Check sheet for the modelled part. Datum: model origin and axes. Units: mm. A direction names the side the tool comes from. Round coordinates to 2 decimals unless told otherwise and drop trailing zeros. Write each loop counter-clockwise with the first axis right and the second up, starting at its lowest first coordinate (ties: lowest second). Pieces come first, ordered by that corner, then holes. Notation, with made-up numbers: (59, 27) -> (75, 27) arc R23 cw to (75, 64) -> close; hole circle Ø6 at (71, 79.5). An arc over 180 degrees is marked (long way). Put each result on its own line as item: value. Start each with the question number.
from build123d import *

# Parameters (mm, degrees)
SKETCH1_W           = 5
SKETCH1_H           = 128.5
BOSS_EXTRUDE1_DEPTH = 2
CUT_EXTRUDE1_DEPTH  = 2.54
FILLET1_R           = 1.27


with BuildPart() as part:
    # Sketch1 → Boss-Extrude1 (new body)
    with BuildSketch(Plane.XY):
        Rectangle(SKETCH1_W, SKETCH1_H)
        with BuildLine():
            Line((-0.254, -59.6), (0.254, -59.6))
            ThreePointArc((0.254, -59.6), (1.904, -61.25), (0.254, -62.9))
            Line((0.254, -62.9), (-0.254, -62.9))
            ThreePointArc((-0.254, -62.9), (-1.904, -61.25), (-0.254, -59.6))
        make_face(mode=Mode.SUBTRACT)
        with BuildLine():
            Line((-0.254, 62.9), (0.254, 62.9))
            ThreePointArc((0.254, 62.9), (1.904, 61.25), (0.254, 59.6))
            Line((0.254, 59.6), (-0.254, 59.6))
            ThreePointArc((-0.254, 59.6), (-1.904, 61.25), (-0.254, 62.9))
        make_face(mode=Mode.SUBTRACT)
    extrude(amount=BOSS_EXTRUDE1_DEPTH)

    # Sketch2 → Cut-Extrude1 (cut)
    with BuildSketch(Plane.XY.offset(2)):
        with BuildLine():
            Line((-0.722, -47.232), (-2.5, -47.232))
            Line((-2.5, -47.232), (-2.5, -50.788))
            Line((-2.5, -50.788), (-0.722, -50.788))
            ThreePointArc((-0.722, -50.788), (1.056, -49.01), (-0.722, -47.232))
        make_face()
    extrude(amount=-CUT_EXTRUDE1_DEPTH, mode=Mode.SUBTRACT)

    # Fillet1
    fillet1_edges = [part.edges().sort_by_distance(p)[0] for p in [
        (-2.5, -47.232, 1),
        (-2.5, -50.788, 1),
    ]]
    fillet(fillet1_edges, radius=FILLET1_R)


solid = part.part
1. Section check A-A, the plane y = 61.25. Enter the section's corners in (x, z).
2. Gauge pin test, flat end, axial feed: P1, Ø1, axis at y = -50.5, z = 1, coming from the -X side. Record the tip position at first contact, or that the pin passes through.
3. Section check B-B, the plane z = 1.05. Enter the section's corners in (x, y).
4. Material ranges on L1, parallel to Y at x = 1.55, z = 0.4; L2, parallel to Y at x = 1.25, z = 0.9; L3, parallel to Y at x = -1.1, z = 0.3, recorded low to high. Write a range as [from, to].
5. Access from +Z, -Z, +X, -X, +Y, -Y to the whole of each face (thin tool, end or side, straight path). Record for faces 1 (the cylindrical face through (1.904, -61.214, 0.986)), 2 (the flat face through (0, 1, 2)).
6. Section check C-C, the plane y = -49.01. Enter the section's corners in (x, z), then the cut area to 3 significant figures.
7. Draft check along Y on faces 3 (the flat face through (0, -64.25, 1)), 4 (the flat face through (0, 1, 0)), 5 (the flat face through (0, 64.25, 1)), 6 (the cylindrical face through (1.904, 61.286, 0.986)). Enter one of: released by +Y, released by -Y, zero draft, split by the parting line, or undercut.
Reply:
1. outline: (-2.5, 0) -> (-1.9, 0) -> (-1.9, 2) -> (-2.5, 2) -> close; (1.9, 0) -> (2.5, 0) -> (2.5, 2) -> (1.9, 2) -> close
2. P1: stops at x = -1.93
3. outline: (-2.5, -64.25) -> (2.5, -64.25) -> (2.5, 64.25) -> (-2.5, 64.25) -> (-2.5, -45.96) arc R1.27 ccw to (-1.23, -47.23) -> (-0.72, -47.23) arc R1.78 cw to (-0.72, -50.79) -> (-1.23, -50.79) arc R1.27 ccw to (-2.5, -52.06) -> close; hole (-0.25, -62.9) -> (0.25, -62.9) arc R1.65 ccw to (0.25, -59.6) -> (-0.25, -59.6) arc R1.65 ccw to start; hole (-0.25, 59.6) -> (0.25, 59.6) arc R1.65 ccw to (0.25, 62.9) -> (-0.25, 62.9) arc R1.65 ccw to start
4. L1: y = [-64.25, -62.27], [-60.23, 60.23], [62.27, 64.25]
4. L2: y = [-64.25, -62.57], [-59.93, 59.93], [62.57, 64.25]
4. L3: y = [-64.25, -62.67], [-59.83, -50.79], [-47.23, 59.83], [62.67, 64.25]
5. face 1: +Z, -Z
5. face 2: +Z, +X, -X, +Y, -Y
6. outline: (1.06, 0) -> (2.5, 0) -> (2.5, 2) -> (1.06, 2) -> close
6. area: 2.89 mm2
7. face 3: released by -Y
7. face 4: zero draft
7. face 5: released by +Y
7. face 6: undercut
